Verification items for the finished model (mm, model axes). A direction names the side the tool comes from. Coordinates: 2 decimals unless noted, no trailing zeros. Write each loop counter-clockwise with the first axis right and the second up, starting at its lowest first coordinate (ties: lowest second). Pieces come first, ordered by that corner, then holes. Notation, with made-up numbers: (17.25, -17) -> (70.25, -17) arc R23 cw to (70.25, 19) -> close; hole circle Ø10 at (45.5, 61). An arc over 180 degrees is marked (long way). Write each question's results on one line, items separated by ' | '. Start each with the question number.
Autodesk Inventor part; units mm, degrees
ref_plane "YZ Plane" through (0, 0, 0) normal (1, 0, 0) x (0, 1, 0)
ref_plane "XZ Plane" through (0, 0, 0) normal (0, 1, 0) x (-1, 0, 0)
ref_plane "XY Plane" through (0, 0, 0) normal (0, 0, 1) x (1, 0, 0)
sketch "スケッチ2" plane through (0, 0, 0) normal (0, 1, 0) x (-1, 0, 0)
  line L0 (-32.5, -11.25) -> (32.5, -11.25)
  line L1 (32.5, -11.25) -> (32.5, 11.25)
  line L2 (32.5, 11.25) -> (-32.5, 11.25)
  line L3 (-32.5, 11.25) -> (-32.5, -11.25)
  line L4 (-32.5, -11.25) -> (32.5, 11.25) construction
  line L5 (32.5, -11.25) -> (-32.5, 11.25) construction
  line L6 (-30, -8.75) -> (30, -8.75)
  line L7 (30, -8.75) -> (30, 8.75)
  line L8 (30, 8.75) -> (-30, 8.75)
  line L9 (-30, 8.75) -> (-30, -8.75)
  line L10 (-30, -8.75) -> (30, 8.75) construction
  line L11 (30, -8.75) -> (-30, 8.75) construction
  circle A0 centre (30, 8.75) radius 2.5
  circle A1 centre (30, -8.75) radius 2.5
  circle A2 centre (-30, 8.75) radius 2.5
  circle A3 centre (-30, -8.75) radius 2.5
  line L12 (-115, -18.25) -> (115, -18.25)
  line L13 (115, -18.25) -> (115, 18.25)
  line L14 (115, 18.25) -> (-115, 18.25)
  line L15 (-115, 18.25) -> (-115, -18.25)
  line L16 (-115, -18.25) -> (115, 18.25) construction
  line L17 (115, -18.25) -> (-115, 18.25) construction
  line L18 (-95, -18.25) -> (95, -18.25)
  line L19 (95, -18.25) -> (95, 18.25)
  line L20 (95, 18.25) -> (-95, 18.25)
  line L21 (-95, 18.25) -> (-95, -18.25)
  line L22 (-95, -18.25) -> (95, 18.25) construction
  line L23 (95, -18.25) -> (-95, 18.25) construction
  point P0 (0, 0)
  dimension "d10" = 65
  dimension "d11" = 22.5
  dimension "d12" = 60
  dimension "d13" = 17.5
  dimension "d14" = 230
  dimension "d15" = 36.5
  dimension "d16" = 190
sketch "スケッチ4" plane through (0, 0, 0) normal (1, 0, 0) x (0, 1, 0)
  point P0 (0, 0)
sketch "スケッチ5" plane through (0, 0, 0) normal (1, 0, 0) x (0, 1, 0)
  circle A0 centre (0, 0) radius 18.25
  line L0 (0, 0) -> (0, 6)
  line L1 (0, 6) -> (0, -6)
  circle A1 centre (0, 6) radius 3
  circle A2 centre (0, -6) radius 9
  circle A3 centre (0, 6) radius 9
  circle A4 centre (0, -6) radius 3
  line L2 (0, 6) -> (5.2915, 0)
  circle A5 centre (5.2915, 0) radius 5
  circle A6 centre (5.2915, 0) radius 4.5
  circle A7 centre (5.2915, 0) radius 5.5
  line L3 (0, 0) -> (0, 11.25)
  line L4 (0, 11.25) -> (0, -11.25)
  line L5 (5.2915, 5.5) -> (5.2915, -5.5)
  line L6 (0, 11.25) -> (-1.2, 11.25)
  line L7 (-1.2, 11.25) -> (-1.2, -11.25)
  line L8 (-1.2, -11.25) -> (0, -11.25)
  line L9 (-1.2, 11.25) -> (-9.2, 11.25)
  line L10 (-1.2, -11.25) -> (-9.2, -11.25)
  line L11 (-9.2, -11.25) -> (-9.2, 11.25)
  line L12 (-9.2, 11.25) -> (-10.4, 11.25)
  line L13 (-10.4, 11.25) -> (-10.4, -11.25)
  line L14 (-10.4, -11.25) -> (-9.2, -11.25)
  circle A8 centre (0, 0) radius 16
  line L15 (0, 11.25) -> (1.5, 11.25)
  line L16 (1.5, 11.25) -> (1.5, -11.25)
  line L17 (1.5, -11.25) -> (0, -11.25)
  line L18 (5.2915, 5.5) -> (1.5, 5.5)
  line L19 (5.2915, -5.5) -> (1.5, -5.5)
  circle A9 centre (5.2915, 0) radius 6.6802
  point P0 (0, 1.5)
  point P1 (0, -1.5)
  point P2 (1.5, -3.9843)
  point P3 (1.5, 3.9843)
  dimension "d28" = 36.5
  dimension "d29" = 6
  dimension "d30" = 12
  dimension "d31" = 6
  dimension "d32" = 18
  dimension "d33" = 8
  dimension "d34" = 9
  dimension "d35" = 11
  dimension "d36" = 11.25
  dimension "d37" = 22.5
  dimension "d39" = 1.2
  dimension "d40" = 8
  dimension "d41" = 1.2
  dimension "d42" = 32
  dimension "d43" = 1.5
ref_plane "作業平面1" through (16.5, 5.2915, 0) normal (1, 0, 0) x (0, 0, 1)
sketch "スケッチ6" plane through (16.5, 5.2915, 0) normal (1, 0, 0) x (0, 0, 1)
  line L0 (0, 5.2915) -> (6, 5.2915)
  line L1 (-11.25, 5.2915) -> (11.25, 5.2915)
  line L2 (6, 5.2915) -> (-6, 5.2915)
  circle A0 centre (6, 5.2915) radius 1.25
  circle A1 centre (-6, 5.2915) radius 1.25
  circle A2 centre (0, 5.2915) radius 16
  circle A3 centre (0, 0) radius 5
  line L3 (0, 0) -> (0, 3)
  line L4 (0, 3) -> (0, -5.5)
  line L5 (0, 3) -> (1, 3)
  line L6 (1, 3) -> (-1, 3)
  line L7 (-1, 3) -> (-1, -5.4083)
  line L8 (1, 3) -> (1, -5.4083)
  circle A4 centre (6, 5.2915) radius 9
  circle A5 centre (-6, 5.2915) radius 9
  line L9 (0, 5.2915) -> (0, -2.7085)
  circle A6 centre (0, -2.7085) radius 8
  circle A7 centre (6, 5.2915) radius 10
  circle A8 centre (-6, 5.2915) radius 10
  line L10 (0, 5.2915) -> (0, -5.7085)
  line L11 (0, -5.7085) -> (-11.619, -5.7085)
  line L12 (0, -5.7085) -> (11.619, -5.7085)
  line L13 (0, -5.7085) -> (9.5, -5.7085)
  line L14 (9.5, -5.7085) -> (-9.5, -5.7085)
  circle A9 centre (0, 5.2915) radius 18
  line L15 (1, -5.4083) -> (1, -8.2085)
  line L16 (-1, -5.4083) -> (-1, -8.2085)
  line L17 (0, 5.2915) -> (0, 6.4915)
  line L18 (0, 6.4915) -> (0, 14.4915)
  line L19 (0, 14.4915) -> (0, 15.6915)
  line L20 (0, 15.6915) -> (-11.25, 15.6915)
  line L21 (-11.25, 15.6915) -> (11.25, 15.6915)
  line L22 (11.25, 15.6915) -> (11.25, 14.4915)
  line L23 (11.25, 14.4915) -> (0, 14.4915)
  line L24 (-11.25, 14.4915) -> (-11.25, 15.6915)
  line L25 (0, 14.4915) -> (-11.25, 14.4915)
  line L26 (0, 15.6915) -> (8.75, 15.6915)
  line L27 (8.75, 15.6915) -> (-8.75, 15.6915)
  line L28 (11.25, 15.6915) -> (11.25, 17.1915)
  line L29 (11.25, 17.1915) -> (-11.25, 17.1915)
  line L30 (-11.25, 17.1915) -> (-11.25, 15.6915)
  line L31 (6, 17.1915) -> (6, 18.6915)
  line L32 (-6, 17.1915) -> (-6, 18.6915)
  circle A10 centre (6, 18.6915) radius 2.5
  circle A11 centre (-6, 18.6915) radius 2.5
  line L33 (6, 21.1915) -> (-6, 21.1915)
  line L34 (9.5, -5.7085) -> (12, -5.7085)
  line L35 (-9.5, -5.7085) -> (-12, -5.7085)
  line L36 (6, 18.6915) -> (8.5, 18.6915)
  line L37 (-6, 18.6915) -> (-8.5, 18.6915)
  circle A12 centre (0, 0) radius 4.5
  circle A13 centre (-6, 5.2915) radius 1.5
  circle A14 centre (6, 5.2915) radius 1.5
  circle A15 centre (6, 18.6915) radius 1.65
  circle A16 centre (-6, 18.6915) radius 1.65
  line L38 (9.5, -5.7085) -> (9.5, -6.2085)
  line L39 (9.5, -6.2085) -> (-9.5, -6.2085)
  line L40 (-9.5, -6.2085) -> (-9.5, -5.7085)
  circle A17 centre (-9.5, -6.2085) radius 1.65
  circle A18 centre (9.5, -6.2085) radius 1.65
  circle A19 centre (9.5, -6.2085) radius 2.5
  circle A20 centre (-9.5, -6.2085) radius 2.5
  line L41 (-12, -6.2085) -> (-8.5, 18.6915)
  line L42 (12, -6.2085) -> (8.5, 18.6915)
  line L43 (9.5, -8.7085) -> (-9.5, -8.7085)
  line L44 (1, -8.7085) -> (1, -8.0358)
  line L45 (-1, -8.7085) -> (-1, -8.2085)
  line L46 (0, 5.2915) -> (-0.3999, 5.2815)
  circle A21 centre (-0.3999, 5.2815) radius 1.7
  line L47 (1.3001, 5.2915) -> (1.3001, -8.7085)
  line L48 (-2.0998, 5.2915) -> (-2.0998, -8.7085)
  line L49 (1.3001, -8.7085) -> (1.1501, -8.7085)
  line L50 (1.1501, -8.7085) -> (1.1501, 4.5832)
  line L51 (-2.0998, -8.7085) -> (-1.9498, -8.7085)
  line L52 (-1.9498, -8.7085) -> (-1.9498, 4.5832)
  line L53 (9.5, -3.7085) -> (-9.5, -3.7085)
  point P0 (1, -4.3875)
  point P1 (-1, -4.3875)
  point P2 (-4.4567, 20.6583)
  point P3 (-8.495, 18.8501)
  point P4 (4.4567, 20.6583)
  point P5 (8.495, 18.8501)
  point P6 (1.7861, 21.1915)
  point P7 (-1.7861, 21.1915)
  point P8 (11.9031, -5.5193)
  point P9 (11.8759, -5.4306)
  point P10 (11.8887, -5.4164)
  point P11 (1.2974, 5.1856)
  point P12 (1.3001, 5.1852)
  point P13 (-11.8759, -5.4306)
  point P14 (-11.0724, -5.7085)
  point P15 (-11.1498, -6.1838)
  point P16 (-11.9297, -5.7085)
  dimension "d54" = 6
  dimension "d55" = 12
  dimension "d56" = 2.5
  dimension "d57" = 2.5
  dimension "d58" = 32
  dimension "d59" = 10
  dimension "d60" = 3
  dimension "d61" = 1
  dimension "d62" = 2
  dimension "d65" = 18
  dimension "d66" = 18
  dimension "d67" = 8
  dimension "d68" = 11
  dimension "d69" = 9.5
  dimension "d70" = 19
  dimension "d73" = 36
  dimension "d76" = 1.2
  dimension "d77" = 8
  dimension "d78" = 1.2
  dimension "d79" = 8.75
  dimension "d80" = 17.5
  dimension "d81" = 1.5
  dimension "d82" = 1.5
  dimension "d83" = 5
  dimension "d84" = 5
  dimension "d97" = 3
  dimension "d98" = 3
  dimension "d109" = 3.3
  dimension "d110" = 3.3
  dimension "d111" = 0.5
  dimension "d112" = 3.3
  dimension "d113" = 3.3
  dimension "d114" = 5
  dimension "d115" = 5
  dimension "d125" = 0.4
  dimension "d126" = 3.4
  dimension "d127" = 0.15
  dimension "d128" = 0.15
extrude "押し出し12" add sketch "スケッチ6" against normal blind 3 contours L50 A12 A21 | A21 A12 L52 | A21 A12 L50 A5 L8 L5 L9 | L9 L6 L7 A4 L52 A12 A21 | L5 L8 A5 L4 L3 | L3 L4 A4 L7 L6 | L50 A8 L8 A5 | A4 L7 A7 L52 | L8 A8 A4 A5 | L50 A4 L8 A8 | A4 A5 A7 L7 | A7 L7 A5 L52 | A4 A8 L4 | L4 A7 A5 | L8 A4 A8 | L50 A7 L8 A4 | A7 A5 L7 | A5 L7 A8 L53 L52 | A7 L8 L53 L4 | A8 L7 A5 A7 | A8 A4 L8 A7 | L4 L53 L7 A8 | L50 L53 L8 A7 | L53 A8 L52 | L53 L8 A12 L4 | L4 A12 L7 L53 | L7 L53 A8 | L50 A12 L8 L53 | A8 L53 L7 A12 L52 | A12 L8 A3 L4 | L4 A3 L7 A12 | L52 A12 L7 A3 | A3 L7 L16 L11 L52 | L50 A3 L8 A12 | L4 L10 L11 L16 L7 A3 | A3 L8 L15 L12 L10 L4 | L50 L12 L15 L8 A3 | L11 L16 L39 L52 | L50 L39 L15 L12 | L11 L12 L15 L39 L16 | L39 L16 L45 L43 L52 | L50 L43 L44 L15 L39 | L39 L15 L44 L43 L45 L16
extrude "押し出し13" add sketch "スケッチ6" along normal blind 2 contours L53 A3 A8 A20 A6 | A6 A20 L53 | L53 A6 A19 A7 A3 | L53 A19 A6 | L53 A12 A8 A3 | A20 A8 A6 | A6 A8 A20 | A3 A7 A12 L53 | A19 A7 A6 | A6 A7 A19 | A8 A6 L11 A17 A2 A20 | A8 A12 L48 A3 | A3 L48 L11 A20 A8 | L53 L48 A8 A12 | A8 A20 L11 A6 | L53 L52 A8 L48 | L53 A8 L52 | L53 L8 A12 L4 | L4 A12 L7 L53 | A7 A19 L12 L47 A3 | A3 L47 A12 A7 | A12 A7 L53 | A19 A2 L12 A18 A6 A7 | A6 L12 A19 A7 | A7 A12 L47 L53 | L47 A12 L50 L53 | A2 L35 L41 A20 | L41 L35 A20 | L48 A12 L52 A3 | A3 L52 L11 L48 | A8 L48 A12 | L11 A20 L39 A6 | A6 L39 A17 L11 | L11 L48 L39 A20 | A8 L52 A12 L48 | L50 A12 L8 L53 | A8 L53 L7 A12 L52 | A12 L8 A3 L4 | L4 A3 L7 A12 | L47 L12 L50 A3 | A3 L50 A12 L47 | A19 L42 L34 A2 | A19 L34 L42 | L12 A18 L39 A6 | A6 L39 A19 L12 | A19 L39 L47 L12 | L11 A17 A2 | A2 A17 A20 L41 L35 | L35 L41 A20 | L52 A12 L7 A3 | A3 L7 L16 L11 L52 | L11 L52 L39 L48 | L39 A20 A6 | A6 A20 A2 A17 L39 | L39 L48 L43 A6 A20 | L50 A3 L8 A12 | L4 L10 L11 L16 L7 A3 | A3 L8 L15 L12 L10 L4 | L50 L12 L15 L8 A3 | L47 L39 L50 L12 | L34 L42 A19 A2 A18 | A2 A18 L12 | A19 L42 L34 | L39 A18 A2 A19 A6 | A6 A19 L39 | A19 A6 L43 L47 L39 | L11 L16 L39 L52 | L39 L52 L43 L48 | A6 L43 A2 A20 | L50 L39 L15 L12 | L47 L43 L50 L39 | A19 A2 L43 A6 | A20 A2 L43 | L11 L12 L15 L39 L16 | L39 L16 L45 L43 L52 | L50 L43 L44 L15 L39 | L43 A2 A19 | L39 L15 L44 L43 L45 L16
properties part number "ikafly1b0.8b"
1. Sectioned sample at A-A on y = 11.5. Record the cut outline in (x, z).
2. Sectioned sample at B-B on z = 9.75. Record the cut outline in (x, y), plus the area to 3 significant figures.
3. Material ranges on probe 1 along Z at (x, y) = (17.85, 11.5); probe 2 along Y at (x, z) = (17.5, 9.5); probe 3 along Z at (x, y) = (14.5, 10), recorded low to high. Write a range as from..to.
4. Tool access check on faces 1 (the flat face through (16.5, 5, 0)), 2 (the flat face through (15, 7, 1.15)), 3 (the flat face through (15, 7, -1.95)). Record the directions out of +Z, -Z, +X, -X, +Y, -Y that give a thin tool (end or side, any length) a straight path to the whole face; none if there is none.
5. Mould release check, pull along Z, two halves, no side actions. Record for faces 4 (the flat face through (17, 9, 0)), 5 (the cylindrical face through (17.5, 11.6, -12)), 6 (the cylindrical face through (17.5, 9.9, -9.9)), 7 (the cylindrical face through (17.5, 9.9, 9.1)): +Z half, -Z half, draft (parallel to the pull), parting line (faces both ways), or undercut.
6. Depth check by flat-ended pin: pin 1 Ø2 at (x, z) = (17.5, 1.5) entering from -Y; pin 2 Ø5.5 at (y, z) = (11, -6.5) entering from -X; pin 3 Ø1.5 at (x, y) = (14.5, 8) entering from -Z; pin 4 Ø1 at (y, z) = (4, 2.5) entering from +X. Enter the tip coordinate at first touch or a pass-through.
7. Sectioned sample at D-D on z = -9.25. Record the cut outline in (x, y), plus the area to 3 significant figures.
8. Sectioned sample at C-C on x = 17.15. Record the cut outline in (y, z).
Computed values:
1) outline: (13.5, -1.95) -> (16.5, -1.95) -> (16.5, -7.85) -> (18.5, -7.85) -> (18.5, 7.85) -> (16.5, 7.85) -> (16.5, 1.15) -> (13.5, 1.15) -> close; (16.5, -12) -> (18.5, -12) -> (18.5, -11.15) -> (16.5, -11.15) -> close; (16.5, 11.15) -> (18.5, 11.15) -> (18.5, 12) -> (16.5, 12) -> close
2) outline: (16.5, 9.01) -> (18.5, 9.01) -> (18.5, 9.87) -> (16.5, 9.87) -> close; (16.5, 13.13) -> (18.5, 13.13) -> (18.5, 13.99) -> (16.5, 13.99) -> close | area: 3.43 mm^2
3) probe 1: z = -12..-11.15, -7.85..7.85, 11.15..12 | probe 2: y = 9..9.85, 13.15..14 | probe 3: z = -1.95..1.15
4) face 1: +Z, -Z, +X, -Y | face 2: +Z, -X, +Y, -Y | face 3: -Z, -X, +Y, -Y
5) face 4: draft | face 5: -Z half | face 6: undercut | face 7: undercut
6) pin 1: stops at y = 9 | pin 2: stops at x = 16.5 | pin 3: stops at z = -1.95 | pin 4: passes through
7) outline: (16.5, 9) -> (18.5, 9) -> (18.5, 9.87) -> (16.5, 9.87) -> close; (16.5, 13.13) -> (18.5, 13.13) -> (18.5, 14) -> (16.5, 14) -> close | area: 3.48 mm^2
8) outline: (9, -9.5) arc R2.5 ccw to (14, -9.5) -> (14, 9.5) arc R2.5 ccw to (9, 9.5) -> close; hole circle Ø3.3 at (11.5, -9.5); hole circle Ø3.3 at (11.5, 9.5)
